Autodesk Inventor part; units mm, degrees
ref_plane "YZ Plane" through (0, 0, 0) normal (1, 0, 0) x (0, 1, 0)
ref_plane "XZ Plane" through (0, 0, 0) normal (0, 1, 0) x (-1, 0, 0)
ref_plane "XY Plane" through (0, 0, 0) normal (0, 0, 1) x (1, 0, 0)
sketch "Sketch1" plane through (0, 0, 0) normal (0, 1, 0) x (-1, 0, 0)
  line L0 (0, 0) -> (80, 0)
  line L1 (80, 0) -> (80, -175)
  line L2 (80, -175) -> (0, -175)
  line L3 (0, -175) -> (0, 0)
  dimension "d0" = 80
  dimension "d1" = 175
extrude "Extrusion1" add sketch "Sketch1" along normal blind 25
sketch "Sketch2" plane through (0, 25, 0) normal (0, 1, 0) x (1, 0, 0)
  point P0 (0, 0)
sketch "Sketch3" plane through (0, 0, 0) normal (1, 0, 0) x (0, 0, -1)
  line L0 (175, 25) -> (0, 25)
  line L1 (160, 25) -> (130, 25)
  line L2 (130, 25) -> (130, 40)
  line L3 (130, 40) -> (160, 40)
  line L4 (160, 40) -> (160, 25)
  line L5 (175, 0) -> (175, 25)
  point P0 (0, 0)
  dimension "d4" = 15
  dimension "d5" = 15
  dimension "d6" = 30
extrude "Extrusion2" add sketch "Sketch3" against normal blind 80
fillet "Fillet1" radius 5 2 edges at (-40, 40, -130) (-40, 40, -160)
sketch "Sketch4" plane through (0, 25, 0) normal (0, 1, 0) x (1, 0, 0)
  circle A0 centre (-63.5, 110) radius 2.5
  circle A1 centre (-20, 110) radius 2.5
  circle A2 centre (-20, 77) radius 2.5
  circle A3 centre (-63.5, 77) radius 2.5
  line L0 (0, 0) -> (0, 130)
  line L1 (-80, 130) -> (0, 130)
  dimension "d10" = 5
  dimension "d11" = 5
  dimension "d12" = 5
  dimension "d13" = 5
  dimension "d14" = 20
  dimension "d15" = 20
  dimension "d16" = 43.5
  dimension "d17" = 43.5
  dimension "d18" = 20
  dimension "d19" = 20
  dimension "d20" = 33
  dimension "d21" = 33
extrude "Extrusion3" add sketch "Sketch4" along normal blind 13
sketch "Sketch5" plane through (-20, 38, -77) normal (0, 1, 0) x (1, 0, 0)
  circle A0 centre (-43.5, 0) radius 2.5
  circle A1 centre (-43.5, 0) radius 1
  circle A2 centre (-43.5, 33) radius 2.5
  circle A3 centre (-43.5, 33) radius 1
  circle A4 centre (0, 33) radius 2.5
  circle A5 centre (0, 33) radius 1
  circle A6 centre (0, 0) radius 2.5
  circle A7 centre (0, 0) radius 1
  point P0 (20, -77)
  dimension "d24" = 2
  dimension "d25" = 2
  dimension "d26" = 2
  dimension "d27" = 2
extrude "Extrusion4" cut sketch "Sketch5" against normal blind 13 contours A1 | A3 | A5 | A7
properties part number "CarApproximation"
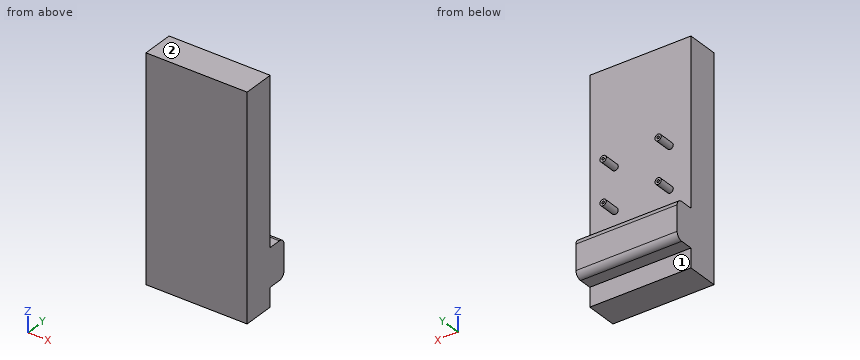
Model file for the job. Use its own axes, mm. Face numbers are marked on the shaded views. A direction names the side the tool comes from. Give positions to 0.01 mm unless a question says otherwise; leave off trailing zeros. Write each loop counter-clockwise with the first axis right and the second up, starting at its lowest first coordinate (ties: lowest second). Pieces come first, ordered by that corner, then holes. Notation, with made-up numbers: (49, -8.5) - (70, -8.5) arc R23 cw to (70, 4.5) - close; hole circle Ø5 at (11.5, 43). An arc over 180 degrees is marked (long way). One line per question, with ' | ' between items. Start each with the question number.
(1) Slice it at B-B on x = -27. Write the cut outline in (y, z).
(2) Wall check: line 1 along Z through (x, y) = (-20, 31.25); line 2 along X through (y, z) = (29.75, -110); line 3 along Z through (x, y) = (-63.5, 35.75). Give the ranges that are in metal, low to high. Write a range as from..to.
(3) Slice it at A-A on y = 27.5. Give the number of separate pieces and of enclosed holes in the cut face, plus the area to 3 significant figures.
(4) Pin check, flat tips, straight feed: P1, Ø1.5, axis at x = -64, z = -109.5, coming from the +Y side; P2, Ø3, axis at x = -70.5, y = 23, coming from the +Z side; P3, Ø0.6, axis at x = -20.5, z = -77, coming from the +Y side; P4, Ø3, axis at x = -35, y = 30.5, coming from the +Z side. Stop position of each tip, or through.
(5) Slice it at C-C on z = -47. Write the cut outline in (x, y), plus the area to 3 significant figures.
(6) 3-axis set-ups, long thin cutter, end or side, ignore diameter. For the marked faces 1 and 2: which of +Z, -Z, +X, -X, +Y, -Y reach the whole face in a straight line?
Results below:
1) outline: (0, -175) - (25, -175) - (25, -160) - (35, -160) arc R5 ccw to (40, -155) - (40, -135) arc R5 ccw to (35, -130) - (25, -130) - (25, 0) - (0, 0) - close
2) line 1: -160..-130, -112.5..-111, -109..-107.5, -79.5..-78, -76..-74.5 | line 2: -66..-64.5, -62.5..-61, -22.5..-21, -19..-17.5 | line 3: -159.94..-130.06, -112.5..-111, -109..-107.5, -79.5..-78, -76..-74.5
3) separate pieces: 5 | enclosed holes: 4 | area: 2,470 mm^2
4) P1: y = 38 | P2: z = 0 | P3: y = 25 | P4: z = -130
5) outline: (-80, 0) - (0, 0) - (0, 25) - (-80, 25) - close | area: 2,000 mm^2
6) face 1: -Z, +X, -X, +Y | face 2: +Z, +X, -X, +Y, -Y
